CAD build for the part. Positions are in the model's coordinates, mm. Face numbers are marked on the shaded views. A direction names the side the tool comes from. Give positions to 0.01 mm unless a question says otherwise; leave off trailing zeros. Order: outer loops, then holes, each group sorted by start corner. A loop starts at its lowest first (then second) coordinate and runs counter-clockwise, first axis right, second up. Notation, with made-up numbers: (81.25, 83.5) -> (89.25, 83.5) arc R8 ccw to (89.25, 93.5) -> close; hole circle Ø9 at (76.25, 23.25). An arc over 180 degrees is marked (long way). Use one line per item in the form item = value. Start each with the question number.
1) Tool access for the marked faces 1 and 2: list every direction of +Z, -Z, +X, -X, +Y, -Y with a clear straight run to the whole face (end or side of a thin tool).
2) Mould opens along X. For the marked faces 3, 4 and 5 say: pulls with the +X half, pulls with the -X half, needs draft (parallel to the pull), parting line crosses it, or undercut.
3) Probe line 1 (X direction, y = -10, z = 16); line 2 (Y direction, x = 5.5, z = 4.5); line 3 (X direction, y = -4, z = 4.25). List the from-to ranges inside material, lowest first.
4) Cut at B-B, the plane y = 11. Give the cut face in (x, z).
5) Cut at C-C, the plane z = 4.25. Give the cut face in (x, y) (3 decimals), and give its area (3 significant figures).
6) Cut at D-D, the plane y = 1. Give the cut face in (x, z).
7) Cut at A-A, the plane x = -4. Give the cut face in (y, z), and give its area (3 significant figures).
8) Drop flat-ended pins along their axis: P1, Ø12, axis at x = -10.5, y = 28, coming from the +Z side; P2, Ø1, axis at x = 0, z = 20.5, coming from the -Y side; P3, Ø0.7, axis at x = -23, y = 27, coming from the +Z side. Give the stop position or say it passes through.
from build123d import *

# Parameters (mm, degrees)
SKETCH_W     = 40
SKETCH_H     = 45
PAD_DEPTH    = 20
SKETCH001_W  = 36
SKETCH001_H  = 46.656231
POCKET_DEPTH = 18
SKETCH002_R  = 1.1
PAD001_DEPTH = 3
SKETCH003_W  = 40
SKETCH003_H  = 10
PAD002_DEPTH = 2
SKETCH004_R  = 1
PAD003_DEPTH = 2


with BuildPart() as part:
    # Sketch → Pad (new body)
    with BuildSketch(Plane.XY):
        with Locations((-8.49515, 10.714768)):
            Rectangle(SKETCH_W, SKETCH_H)
    extrude(amount=PAD_DEPTH)

    # Sketch001 → Pocket (cut)
    with BuildSketch(Plane.XY.offset(20)):
        with Locations((-8.49515, 7.886653)):
            Rectangle(SKETCH001_W, SKETCH001_H)
    extrude(amount=-POCKET_DEPTH, mode=Mode.SUBTRACT)

    # Sketch002 → Pad001 (new body)
    with BuildSketch(Plane.XY.offset(2)):
        with Locations((-22.475006, 27.009532)):
            Circle(SKETCH002_R)
        with Locations((5.464994, -4.740468)):
            Circle(SKETCH002_R)
    extrude(amount=PAD001_DEPTH)

    # Sketch003 → Pad002 (new body)
    with BuildSketch(Plane.XY.offset(20)):
        with Locations((-8.49515, 15.142302)):
            Rectangle(SKETCH003_W, SKETCH003_H)
    extrude(amount=PAD002_DEPTH)

    # Sketch004 → Pad003 (new body)
    with BuildSketch(Plane.XY.offset(22)):
        with Locations((-23.518098, 15.142302)):
            Circle(SKETCH004_R)
        with Locations((6.481902, 15.142302)):
            Circle(SKETCH004_R)
    extrude(amount=PAD003_DEPTH)


solid = part.part
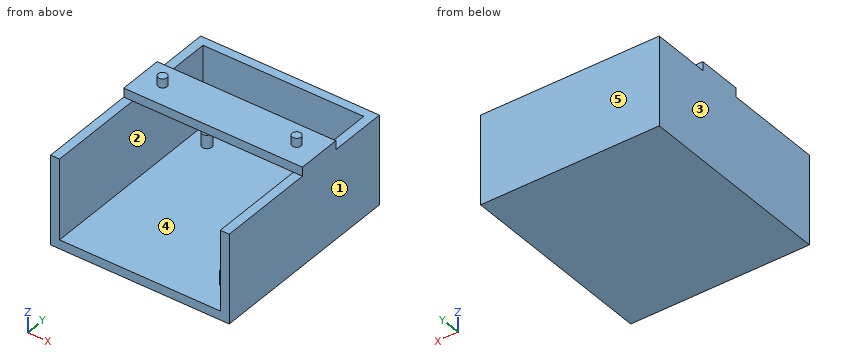
Result:
q1.face_1 = +Z, -Z, +X, +Y, -Y
q1.face_2 = -Y
q2.face_3 = pulls with the -X half
q2.face_4 = undercut
q2.face_5 = needs draft
q3.line_1 = -28.5 to -26.5, 9.5 to 11.5
q3.line_2 = -5.84 to -3.64, 31.21 to 33.21
q3.line_3 = -28.5 to -26.5, 4.65 to 6.28, 9.5 to 11.5
q4.outline = (-28.5, 0) -> (11.5, 0) -> (11.5, 22) -> (-28.5, 22) -> close; hole (-26.5, 2) -> (9.5, 2) -> (9.5, 20) -> (-26.5, 20) -> close
q5.outline = (-28.495, -11.785) -> (-26.495, -11.785) -> (-26.495, 31.215) -> (9.505, 31.215) -> (9.505, -11.785) -> (11.505, -11.785) -> (11.505, 33.215) -> (-28.495, 33.215) -> close; circle Ø2.2 at (-22.475, 27.01); circle Ø2.2 at (5.465, -4.74)
q5.area = 260 mm²
q6.outline = (-28.5, 0) -> (11.5, 0) -> (11.5, 20) -> (9.5, 20) -> (9.5, 2) -> (-26.5, 2) -> (-26.5, 20) -> (-28.5, 20) -> close
q7.outline = (-11.79, 0) -> (33.21, 0) -> (33.21, 20) -> (31.21, 20) -> (31.21, 2) -> (-11.79, 2) -> close; (10.14, 20) -> (20.14, 20) -> (20.14, 22) -> (10.14, 22) -> close
q7.area = 146 mm²
q8.P1 = 20
q8.P2 = 10.14
q8.P3 = 5
